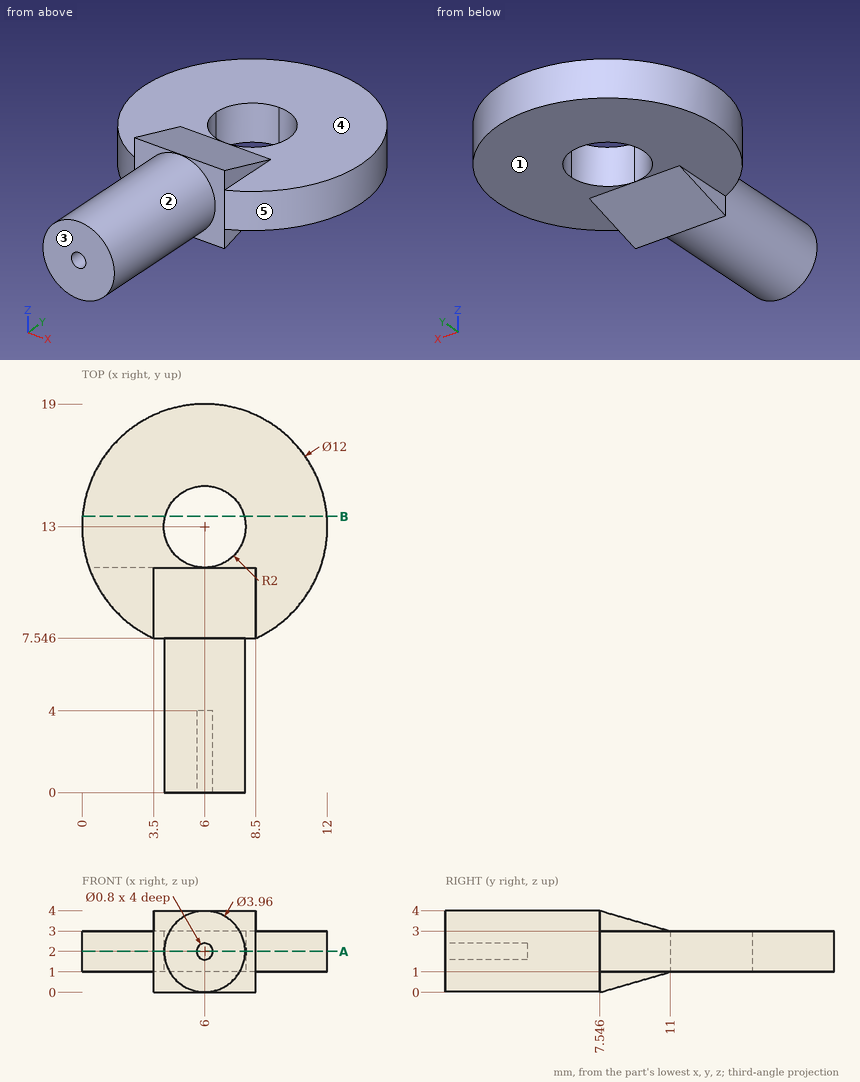
Input: dimensioned drawing with shaded views. Units: mm. Origin: part minimum x, y, z. A direction names the side the tool comes from. Give positions to 0.01 mm unless a question says otherwise; leave off trailing zeros. Write each loop counter-clockwise with the first axis right and the second up, starting at its lowest first coordinate (ties: lowest second). Pieces come first, ordered by that corner, then holes. Notation, with made-up numbers: (42, -5) - (98, -5) arc R30 ccw to (98, 18) - close; hole circle Ø3 at (-34.75, 47.25). An arc over 180 degrees is marked (long way). Write item = value, one per line. Start each with the question number.
1) Cut plane B-B (y = 13.5). Return loops of the section in (x, z).
2) Pin query (flat end, axial travel): pin 1 (1 mm diameter, centred on x = 9, z = 2, fed in from +Y) (1 decimal); pin 2 (3.5 mm diameter, centred on x = 5, y = 12.5, fed in from -Z). Return the tip coordinate at first contact, or that it passes through.
3) Material intervals for L1, parallel to Z at x = 6, y = 1.6; L2, parallel to X at y = 9, z = 3.1; L3, parallel to X at y = 3, z = 1.8 (1 decimal), sorted ascending. Write a range as [from, to].
4) Reachability of the marked faces 1, 2, 3, 4 and 5 from +Z, -Z, +X, -X, +Y, -Y: full face, straight path, thin tool, end or side. Return the list, or none.
5) Cut plane A-A (z = 2). Return loops of the section in (x, y) (1 decimal), and give its area (3 significant figures).
Answers follow:
q1.outline = (0.02, 1) - (4.06, 1) - (4.06, 3) - (0.02, 3) - close; (7.94, 1) - (11.98, 1) - (11.98, 3) - (7.94, 3) - close
q2.pin_1 = 18.5
q2.pin_2 = 0.93
q3.L1 = [0.02, 1.6], [2.4, 3.98]
q3.L2 = [3.5, 8.5]
q3.L3 = [4, 5.7], [6.3, 8]
q4.face_1 = -Z, +Y
q4.face_2 = -Y
q4.face_3 = +Z, -Z, +X, -X, -Y
q4.face_4 = +Z, +Y
q4.face_5 = +Z, -Z
q5.outline = (3.5, 7.5) - (4, 7.5) - (4, 0) - (5.6, 0) - (5.6, 4) - (6.4, 4) - (6.4, 0) - (8, 0) - (8, 7.5) - (8.5, 7.5) arc R6 ccw (long way) to start; hole circle Ø4 at (6, 13)
q5.area = 125 mm^2
